from build123d import *

# Parameters (mm, degrees)
PAD_DEPTH       = 10
SKETCH001_W     = 9.110509
SKETCH001_H     = 17.177114
POCKET_DEPTH    = 3.001
SKETCH002_R     = 1.4
POCKET001_DEPTH = 2.048058
FILLET_R        = 0.25


with BuildPart() as part:
    # Sketch → Pad (new body)
    with BuildSketch(Plane.XY):
        with BuildLine():
            Line((25, 0), (25, -12.5))
            ThreePointArc((23, -14.5), (24.414214, -13.914214), (25, -12.5))
            Line((23, -14.5), (19, -14.5))
            ThreePointArc((18, -13.5), (18.292893, -14.207107), (19, -14.5))
            Line((18, -13.5), (18, -11.5))
            Line((18, -11.5), (21, -11.5))
            Line((21, -11.5), (21, -1))
            Line((21, -1), (-21, -1))
            Line((-21, -1), (-21, -11.5))
            Line((-21, -11.5), (-18, -11.5))
            Line((-18, -11.5), (-18, -13.5))
            ThreePointArc((-19, -14.5), (-18.292893, -14.207107), (-18, -13.5))
            Line((-19, -14.5), (-22.634118, -14.5))
            ThreePointArc((-24, -13.960947), (-23.36832, -14.360362), (-22.634118, -14.5))
            Line((-24, -13.960947), (-24, -2.048058))
            Line((-24, -2.048058), (-34.206213, -2.048058))
            Line((-34.206213, -2.048058), (-34.206213, 0))
            Line((-34.206213, 0), (-21, 0))
            Line((-21, 0), (21, 0))
            ThreePointArc((21, 0), (0.10979, 5.111176), (-21, 1))
            Line((-21, 1), (-34.206213, 1))
            Line((-34.206213, 1), (-34.206213, 3.048058))
            Line((-34.206213, 3.048058), (-21, 3.048058))
            ThreePointArc((25, 0), (2.356054, 6.897451), (-21, 3.048058))
        make_face()
    extrude(amount=PAD_DEPTH)

    # Sketch001 (on Face16 of Pad) → Pocket (cut, through all)
    with BuildSketch(Plane(origin=(0, -11.5, 0), x_dir=(-1, 0, 0), z_dir=(0, 1, 0))):
        with Locations((-4.555255, 16.023105)):
            Rectangle(SKETCH001_W, SKETCH001_H)
    extrude(amount=-POCKET_DEPTH, mode=Mode.SUBTRACT)

    # Sketch002 (on Face2 of Pad) → Pocket001 (cut)
    with BuildSketch(Plane.XZ.offset(2.048058)):
        with Locations((-29.103106, 5)):
            Circle(SKETCH002_R)
    extrude(amount=-POCKET001_DEPTH, mode=Mode.SUBTRACT)

    # Fillet
    fillet_edges = [part.edges().sort_by_distance(p)[0] for p in [
        (-24, -8.004502, 0),
        (-29.103106, -2.048058, 0),
        (-34.206213, -1.024029, 0),
        (-27.603106, 0, 0),
        (0, 0, 0),
        (0.10979, 5.111176, 0),
        (-27.603106, 1, 0),
        (-34.206213, 2.024029, 0),
        (-27.603106, 3.048058, 0),
        (2.356054, 6.897451, 0),
        (25, -6.25, 0),
        (24.414214, -13.914214, 0),
        (21, -14.5, 0),
        (18.292893, -14.207107, 0),
        (18, -12.5, 0),
        (19.5, -11.5, 0),
        (21, -6.25, 0),
        (0, -1, 0),
        (-21, -6.25, 0),
        (-19.5, -11.5, 0),
        (-18, -12.5, 0),
        (-18.292893, -14.207107, 0),
        (-20.817059, -14.5, 0),
        (-23.36832, -14.360362, 0),
        (-24, -8.004502, 10),
        (-29.103106, -2.048058, 10),
        (-34.206213, -1.024029, 10),
        (-27.603106, 0, 10),
        (0, 0, 10),
        (0.10979, 5.111176, 10),
        (-27.603106, 1, 10),
        (-34.206213, 2.024029, 10),
        (-27.603106, 3.048058, 10),
        (2.356054, 6.897451, 10),
        (25, -6.25, 10),
        (24.414214, -13.914214, 10),
        (21, -14.5, 10),
        (18.292893, -14.207107, 10),
        (18, -12.5, 10),
        (19.5, -11.5, 10),
        (21, -6.25, 10),
        (0, -1, 10),
        (-21, -6.25, 10),
        (-19.5, -11.5, 10),
        (-18, -12.5, 10),
        (-18.292893, -14.207107, 10),
        (-20.817059, -14.5, 10),
        (-23.36832, -14.360362, 10),
    ]]
    fillet(fillet_edges, radius=FILLET_R)


solid = part.part
Build history of the part. All positions in model axes, mm. A direction names the side the tool comes from. Coordinates: 2 decimals unless noted, no trailing zeros. Write each loop counter-clockwise with the first axis right and the second up, starting at its lowest first coordinate (ties: lowest second). Pieces come first, ordered by that corner, then holes.
(1) Mould opens along Y. For faces 5 (the flat face through (-18, -12, 5)), 6 (the cylindrical face through (18.285, -14.199, 4.934)), 7 (the flat face through (-20, -11.5, 5)) say: pulls with the +Y half, pulls with the -Y half, needs draft (parallel to the pull), parting line crosses it, or undercut.
(2) Pin check, flat tips, straight feed: pin 1 Ø1.6 at (y, z) = (-12, 3.5) entering from -X; pin 2 Ø3.5 at (x, z) = (-19.5, 5) entering from +Y; pin 3 Ø3 at (x, z) = (-14, 3) entering from +Y. Stop position of each tip, or through.
(3) Cut at A-A on z = 5. List the corners of the cut face in (x, y).
(4) Drill centre lines: line 1 (X direction, y = -2, z = 1); line 2 (Y direction, x = 18.5, z = 4.75); line 3 (X direction, y = -9.5, z = 2.5). Where is each one in solid material? Low to high.
(5) Cut at B-B on y = -8.25. List the corners of the cut face in (x, z), and give its area (3 significant figures).
(6) 3-axis set-ups, long thin cutter, end or side, ignore diameter. For faces 1 (the flat face through (0, -1, 5)), 2 (the flat face through (-28, 3.048, 5)), 3 (the cylindrical face through (-30.5, -1, 5.1)), 4 (the flat face through (18, -13, 5)): which of +Z, -Z, +X, -X, +Y, -Y reach the whole face in a straight line?
Working result:
1. face 5: needs draft
1. face 6: pulls with the -Y half
1. face 7: undercut
2. pin 1: stops at x = -24
2. pin 2: stops at y = 4.27
2. pin 3: stops at y = 5.74
3. outline: (-34.21, -2.05) - (-30.5, -2.05) - (-30.5, 0) - (-34.21, 0) - close; (-34.21, 1) - (-21, 1) arc R50.14 cw to (21, 0) - (-27.7, 0) - (-27.7, -2.05) - (-24, -2.05) - (-24, -13.96) arc R2 ccw to (-22.63, -14.5) - (-19, -14.5) arc R1 ccw to (-18, -13.5) - (-18, -11.5) - (-21, -11.5) - (-21, -1) - (21, -1) - (21, -11.5) - (18, -11.5) - (18, -13.5) arc R1 ccw to (19, -14.5) - (23, -14.5) arc R2 ccw to (25, -12.5) - (25, 0) arc R52.02 ccw to (-21, 3.05) - (-34.21, 3.05) - close
4. line 1: x = -34.21 to -21, 21 to 25
4. line 2: y = -14.37 to -11.5, -1 to 0, 1.14 to 3.18
4. line 3: x = -24 to -21, 21 to 25
5. outline: (-24, 0.25) arc R0.25 ccw to (-23.75, 0) - (-21.25, 0) arc R0.25 ccw to (-21, 0.25) - (-21, 9.75) arc R0.25 ccw to (-21.25, 10) - (-23.75, 10) arc R0.25 ccw to (-24, 9.75) - close; (21, 0.25) arc R0.25 ccw to (21.25, 0) - (24.75, 0) arc R0.25 ccw to (25, 0.25) - (25, 9.75) arc R0.25 ccw to (24.75, 10) - (21.25, 10) arc R0.25 ccw to (21, 9.75) - close
5. area: 69.9 mm2
6. face 1: +Z, -Z
6. face 2: +Z, -Z, -X, +Y
6. face 3: -Y
6. face 4: +Z, -Z, -Y
